The listing builds one solid part. Answer for the finished solid, in the listing's coordinates (mm). Coordinates: 2 decimals unless noted, no trailing zeros. Return JSON: item names as keys, results as strings.
from build123d import *

# Parameters (mm, degrees)
SKETCH11_R          = 1
SKETCH11_R_2        = 2.1
XA_XA_2020T_1_DEPTH = 400
SKETCH14_W          = 25.965356462
SKETCH14_H          = 24.672555304
CUT_EXTRUDE2_DEPTH  = 30


with BuildPart() as part:
    # Sketch11 → Xa XA-2020T(1) (new body)
    with BuildSketch(Plane(origin=(0, 0, 0), x_dir=(0, 0, -1), z_dir=(1, 0, 0))):
        with BuildLine():
            Line((-9.889124212, 8.439448346), (-9.889124212, 3.289448346))
            ThreePointArc((-9.889124212, 3.289448346), (-9.815900907, 3.112671651), (-9.639124212, 3.039448346))
            Line((-9.639124212, 3.039448346), (-7.889124212, 3.039448346))
            Line((-7.889124212, 3.039448346), (-7.889124212, 5.039448346))
            Line((-7.889124212, 5.039448346), (-6.41690199, 5.039448346))
            Line((-6.41690199, 5.039448346), (-3.889124212, 2.439448346))
            Line((-3.889124212, 2.439448346), (-3.889124212, -2.560551654))
            Line((-3.889124212, -2.560551654), (-6.41690199, -5.160551654))
            Line((-6.41690199, -5.160551654), (-7.889124212, -5.160551654))
            Line((-7.889124212, -5.160551654), (-7.889124212, -3.160551654))
            Line((-7.889124212, -3.160551654), (-9.639124212, -3.160551654))
            ThreePointArc((-9.639124212, -3.160551654), (-9.815900907, -3.233774958), (-9.889124212, -3.410551654))
            Line((-9.889124212, -3.410551654), (-9.889124212, -8.560551654))
            ThreePointArc((-9.889124212, -8.560551654), (-9.449784384, -9.621211825), (-8.389124212, -10.060551654))
            Line((-8.389124212, -10.060551654), (-3.239124212, -10.060551654))
            ThreePointArc((-3.239124212, -10.060551654), (-3.062347516, -9.987328349), (-2.989124212, -9.810551654))
            Line((-2.989124212, -9.810551654), (-2.989124212, -8.060551654))
            Line((-2.989124212, -8.060551654), (-4.989124212, -8.060551654))
            Line((-4.989124212, -8.060551654), (-4.989124212, -6.588329431))
            Line((-4.989124212, -6.588329431), (-2.389124212, -4.060551654))
            Line((-2.389124212, -4.060551654), (2.610875788, -4.060551654))
            Line((2.610875788, -4.060551654), (5.210875788, -6.588329431))
            Line((5.210875788, -6.588329431), (5.210875788, -8.060551654))
            Line((5.210875788, -8.060551654), (3.210875788, -8.060551654))
            Line((3.210875788, -8.060551654), (3.210875788, -9.810551654))
            ThreePointArc((3.210875788, -9.810551654), (3.284099093, -9.987328349), (3.460875788, -10.060551654))
            Line((3.460875788, -10.060551654), (8.610875788, -10.060551654))
            ThreePointArc((8.610875788, -10.060551654), (9.67153596, -9.621211825), (10.110875788, -8.560551654))
            Line((10.110875788, -8.560551654), (10.110875788, -3.410551654))
            ThreePointArc((10.110875788, -3.410551654), (10.037652484, -3.233774958), (9.860875788, -3.160551654))
            Line((9.860875788, -3.160551654), (8.110875788, -3.160551654))
            Line((8.110875788, -3.160551654), (8.110875788, -5.160551654))
            Line((8.110875788, -5.160551654), (6.638653566, -5.160551654))
            Line((6.638653566, -5.160551654), (4.110875788, -2.560551654))
            Line((4.110875788, -2.560551654), (4.110875788, 2.439448346))
            Line((4.110875788, 2.439448346), (6.638653566, 5.039448346))
            Line((6.638653566, 5.039448346), (8.110875788, 5.039448346))
            Line((8.110875788, 5.039448346), (8.110875788, 3.039448346))
            Line((8.110875788, 3.039448346), (9.860875788, 3.039448346))
            ThreePointArc((9.860875788, 3.039448346), (10.037652484, 3.112671651), (10.110875788, 3.289448346))
            Line((10.110875788, 3.289448346), (10.110875788, 8.439448346))
            ThreePointArc((10.110875788, 8.439448346), (9.67153596, 9.500108518), (8.610875788, 9.939448346))
            Line((8.610875788, 9.939448346), (3.460875788, 9.939448346))
            ThreePointArc((3.460875788, 9.939448346), (3.284099093, 9.866225042), (3.210875788, 9.689448346))
            Line((3.210875788, 9.689448346), (3.210875788, 7.939448346))
            Line((3.210875788, 7.939448346), (5.210875788, 7.939448346))
            Line((5.210875788, 7.939448346), (5.210875788, 6.467226124))
            Line((5.210875788, 6.467226124), (2.610875788, 3.939448346))
            Line((2.610875788, 3.939448346), (-2.389124212, 3.939448346))
            Line((-2.389124212, 3.939448346), (-4.989124212, 6.467226124))
            Line((-4.989124212, 6.467226124), (-4.989124212, 7.939448346))
            Line((-4.989124212, 7.939448346), (-2.989124212, 7.939448346))
            Line((-2.989124212, 7.939448346), (-2.989124212, 9.689448346))
            ThreePointArc((-2.989124212, 9.689448346), (-3.062347516, 9.866225042), (-3.239124212, 9.939448346))
            Line((-3.239124212, 9.939448346), (-8.389124212, 9.939448346))
            ThreePointArc((-8.389124212, 9.939448346), (-9.449784384, 9.500108518), (-9.889124212, 8.439448346))
        make_face()
        with Locations((-7.439124212, 7.489448346)):
            Circle(SKETCH11_R, mode=Mode.SUBTRACT)
        with Locations((7.660875788, 7.489448346)):
            Circle(SKETCH11_R, mode=Mode.SUBTRACT)
        with Locations((-7.439124212, -7.610551654)):
            Circle(SKETCH11_R, mode=Mode.SUBTRACT)
        with Locations((7.660875788, -7.610551654)):
            Circle(SKETCH11_R, mode=Mode.SUBTRACT)
        Circle(SKETCH11_R_2, mode=Mode.SUBTRACT)
    extrude(amount=XA_XA_2020T_1_DEPTH)

    # Sketch14 → Cut-Extrude2 (cut)
    with BuildSketch(Plane(origin=(400, 0, 0), x_dir=(0, 0, -1), z_dir=(1, 0, 0))):
        Rectangle(SKETCH14_W, SKETCH14_H)
    extrude(amount=-CUT_EXTRUDE2_DEPTH, mode=Mode.SUBTRACT)


solid = part.part
1. The part is cut by section A-A on x = 72.5. Give the number of separate pieces and of enclosed holes in the cut face, and give its area (3 significant figures).
Answer block:
{"separate pieces": "1", "enclosed holes": "5", "area": "185 mm2"}
2. Consider line 1 (Y direction, x = 68.5, z = 7.25); line 2 (Y direction, x = 23, z = -3.75); line 3 (Z direction, x = 17.5, y = 3.5). Determine where each line is inside the solid, lowest interval first. Write a range as from..to.
Answer block:
{"line 1": "y = -10.06..-8.59, -6.63..-5.16, 5.04..6.51, 8.47..9.94", "line 2": "y = -10.06..-8.06, -5.17..5.05, 7.94..9.94", "line 3": "z = -10.11..-8.11, -5.14..4.92, 7.89..9.89"}
3. Each of these flat-tipped pins is pushed along its axis until it touches: pin 1 Ø1 at (x, y) = (211.5, 0.5) entering from +Z; pin 2 Ø1.5 at (x, z) = (180.5, -0.5) entering from +Y; pin 3 Ø1.5 at (x, z) = (197, 0.5) entering from -Y. Where does it stop, or does it pass through?
Answer block:
{"pin 1": "stops at z = 3.89", "pin 2": "stops at y = 3.94", "pin 3": "stops at y = -4.06"}
